The model under review builds one solid part; all positions refer to its coordinate system, in mm. A direction names the side the tool comes from. Round coordinates to 2 decimals unless told otherwise and drop trailing zeros. Loops run counter-clockwise (first coordinate to the right, second up) from the corner with the lowest first, then second, coordinate; pieces in that order, holes last. Notation, with made-up numbers: (-9, 75) -> (18, 75) arc R12 ccw to (18, 94) -> close; hole circle Ø10 at (-21, 69). An arc over 180 degrees is marked (long way). Write each question's results on one line, items separated by ' | '. Start each with the question number.
Item 1: Tool access review of faces 1 (the flat face through (22.272, 24, 5)), 2 (the flat face through (-17, 5.702, 5)): name each direction out of +Z, -Z, +X, -X, +Y, -Y from which nothing blocks a thin tool from reaching the whole face with its end or side.
Item 2: We need section B-B (y = -21.5). Give the boundary of the cut face in (x, z), and give its area (3 significant figures).
Item 3: We need section C-C (z = 1.25). Give the boundary of the cut face in (x, y), and give its area (3 significant figures).
Item 4: Mouldability with a two-part tool opening along X and no side actions: class faces 3 (the flat face through (-57.728, 24, 5)), 4 (the cylindrical face through (-47.7, -24.8, 4.9)), 5 (the flat face through (-18, -32.798, 5)), 6 (the cylindrical face through (-49.228, 27.169, 4.93)) as pulls with the +X half, pulls with the -X half, needs draft (parallel to the pull), parting line crosses it, or undercut.
Item 5: We need section A-A (x = 3). Give the boundary of the cut face in (y, z).
Item 6: For L1, parallel to Y at x = 9, z = 1; L2, parallel to X at y = -9, z = 1; L3, parallel to Y at x = -49, z = 1, list the stretches that pass through material, from the lowest coordinate up. Write a range as from..to.
from build123d import *

# Parameters (mm, degrees)
ESQUISSE1_W        = 80
ESQUISSE1_H        = 115
ESQUISSE1_R        = 1.5
BOSS_EXTRU_1_DEPTH = 10


with BuildPart() as part:
    # Esquisse1 → Boss.-Extru.1 (new body)
    with BuildSketch(Plane.XY):
        with Locations((-17.727954042, 24.701649019)):
            Rectangle(ESQUISSE1_W, ESQUISSE1_H)
        with Locations((-47.727954042, 77.201649019)):
            Circle(ESQUISSE1_R, mode=Mode.SUBTRACT)
        with Locations((12.272045958, 77.201649019)):
            Circle(ESQUISSE1_R, mode=Mode.SUBTRACT)
        with BuildLine():
            Line((-47.727954042, 28.701649019), (12.272045958, 28.701649019))
            ThreePointArc((12.272045958, 28.701649019), (13.772045958, 27.201649019), (12.272045958, 25.701649019))
            Line((12.272045958, 25.701649019), (-47.727954042, 25.701649019))
            ThreePointArc((-47.727954042, 25.701649019), (-49.227954042, 27.201649019), (-47.727954042, 28.701649019))
        make_face(mode=Mode.SUBTRACT)
        with BuildLine():
            Line((-47.727954042, 8.701649019), (12.272045958, 8.701649019))
            ThreePointArc((12.272045958, 8.701649019), (13.772045958, 7.201649019), (12.272045958, 5.701649019))
            Line((12.272045958, 5.701649019), (-47.727954042, 5.701649019))
            ThreePointArc((-47.727954042, 5.701649019), (-49.227954042, 7.201649019), (-47.727954042, 8.701649019))
        make_face(mode=Mode.SUBTRACT)
        with BuildLine():
            Line((-49.727954042, -22.798350981), (-49.727954042, -2.798350981))
            ThreePointArc((-49.727954042, -2.798350981), (-47.727954042, -0.798350981), (-45.727954042, -2.798350981))
            Line((-45.727954042, -2.798350981), (-45.727954042, -22.798350981))
            ThreePointArc((-45.727954042, -22.798350981), (-47.727954042, -24.798350981), (-49.727954042, -22.798350981))
        make_face(mode=Mode.SUBTRACT)
        with BuildLine():
            Line((10.272045958, -2.798350981), (10.272045958, -22.798350981))
            ThreePointArc((10.272045958, -22.798350981), (12.272045958, -24.798350981), (14.272045958, -22.798350981))
            Line((14.272045958, -22.798350981), (14.272045958, -2.798350981))
            ThreePointArc((14.272045958, -2.798350981), (12.272045958, -0.798350981), (10.272045958, -2.798350981))
        make_face(mode=Mode.SUBTRACT)
    extrude(amount=BOSS_EXTRU_1_DEPTH)


solid = part.part
Here are the results:
1) face 1: +Z, -Z, +X, +Y, -Y | face 2: +Z, -Z
2) outline: (-57.73, 0) -> (-49.73, 0) -> (-49.73, 10) -> (-57.73, 10) -> close; (-45.73, 0) -> (10.27, 0) -> (10.27, 10) -> (-45.73, 10) -> close; (14.27, 0) -> (22.27, 0) -> (22.27, 10) -> (14.27, 10) -> close | area: 720 mm2
3) outline: (-57.73, -32.8) -> (22.27, -32.8) -> (22.27, 82.2) -> (-57.73, 82.2) -> close; hole (-49.73, -22.8) arc R2 ccw to (-45.73, -22.8) -> (-45.73, -2.8) arc R2 ccw to (-49.73, -2.8) -> close; hole circle Ø3 at (-47.73, 77.2); hole (-47.73, 5.7) -> (12.27, 5.7) arc R1.5 ccw to (12.27, 8.7) -> (-47.73, 8.7) arc R1.5 ccw to start; hole (-47.73, 25.7) -> (12.27, 25.7) arc R1.5 ccw to (12.27, 28.7) -> (-47.73, 28.7) arc R1.5 ccw to start; hole (10.27, -22.8) arc R2 ccw to (14.27, -22.8) -> (14.27, -2.8) arc R2 ccw to (10.27, -2.8) -> close; hole circle Ø3 at (12.27, 77.2) | area: 8,630 mm2
4) face 3: pulls with the -X half | face 4: undercut | face 5: needs draft | face 6: undercut
5) outline: (-32.8, 0) -> (5.7, 0) -> (5.7, 10) -> (-32.8, 10) -> close; (8.7, 0) -> (25.7, 0) -> (25.7, 10) -> (8.7, 10) -> close; (28.7, 0) -> (82.2, 0) -> (82.2, 10) -> (28.7, 10) -> close
6) L1: y = -32.8..5.7, 8.7..25.7, 28.7..82.2 | L2: x = -57.73..-49.73, -45.73..10.27, 14.27..22.27 | L3: y = -32.8..-24.34, -1.26..6.41, 8..26.41, 28..76.41, 78..82.2
